The model under review builds one solid part; all positions refer to its coordinate system, in mm. Round coordinates to 2 decimals unless told otherwise and drop trailing zeros. Write each loop counter-clockwise with the first axis right and the second up, starting at its lowest first coordinate (ties: lowest second). Pieces come first, ordered by that corner, then holes.
Item 1: Add section D-D (z = 4.25). Give the boundary of the cut face in (x, y), plus the area to 3 significant figures.
Item 2: Draft analysis for pull direction Y (two halves, no side actions). For faces 1 (the face through (-0.867, -3.905, -2.104)), 2 (the face through (0.61, -2.74, -0.18)), 3 (the face through (2.2, -2.2, 12.7)), state which applies: +Y half, -Y half, draft (parallel to the pull), parting line (faces both ways), or undercut.
Item 3: Add section A-A (y = 0). Give the boundary of the cut face in (x, z) (3 decimals).
Item 4: Clearance check with flat-ended pins moving along their axes: pin 1 Ø1.5 at (y, z) = (4, -7.5) entering from -X; pin 2 Ø4 at (y, z) = (3.5, 2) entering from +X; pin 3 Ø5 at (x, z) = (0.5, 0.5) entering from +Y. State where each tip first meets the part, or that it passes through.
Item 5: To check wall thickness, follow L1, parallel to Y at x = 0, z = 1.5; L2, parallel to Y at x = -2, z = 4.75; L3, parallel to Z at x = 2.75, y = 3.5. State the ranges of each line that lie inside material, in increasing order.
Item 6: Add section C-C (z = 9). Give the boundary of the cut face in (x, y) (3 decimals), plus the area to 3 significant figures.
```python
from build123d import *

# Parameters (mm, degrees)
SKETCH1_R              = 4
BOSS_EXTRUDE1_DEPTH    = 12.7
F_10_CLEARANCE_HOLE1_D = 5.6134
BOSS_EXTRUDE2_START    = -4
SKETCH4_R              = 5.125
SKETCH4_R_2            = 2.8067
BOSS_EXTRUDE2_DEPTH    = 4
FILLET1_R              = 0.5


with BuildPart() as part:
    # Sketch1 → Boss-Extrude1 (new, symmetric)
    with BuildSketch(Plane.XY):
        Circle(SKETCH1_R)
    extrude(amount=BOSS_EXTRUDE1_DEPTH, both=True)

    # #10 Clearance Hole1 (through all)
    with Locations(Plane.XY.offset(12.7)):
        with Locations((0, 0)):
            Hole(F_10_CLEARANCE_HOLE1_D / 2)

    # Sketch4 → Boss-Extrude2 (add)
    with BuildSketch(Plane.XY.offset(12.7).offset(BOSS_EXTRUDE2_START)):
        Circle(SKETCH4_R)
        Circle(SKETCH4_R_2, mode=Mode.SUBTRACT)
    extrude(amount=BOSS_EXTRUDE2_DEPTH)

    # Fillet1
    fillet1_edges = [part.edges().sort_by_distance(p)[0] for p in [
        (-4, 0, 8.7),
    ]]
    fillet(fillet1_edges, radius=FILLET1_R)


solid = part.part
```
Numbers:
1. outline: circle Ø8 at (0, 0); hole circle Ø5.61 at (0, 0)
1. area: 25.5 mm2
2. face 1: parting line
2. face 2: undercut
2. face 3: draft
3. outline: (-5.125, 8.7) - (-4.5, 8.7) arc R0.5 cw to (-4, 8.2) - (-4, -12.7) - (-2.807, -12.7) - (-2.807, 12.7) - (-5.125, 12.7) - close; (2.807, -12.7) - (4, -12.7) - (4, 8.2) arc R0.5 cw to (4.5, 8.7) - (5.125, 8.7) - (5.125, 12.7) - (2.807, 12.7) - close
4. pin 1: stops at x = -2.33
4. pin 2: stops at x = 3.71
4. pin 3: stops at y = 4
5. L1: y = -4 to -2.81, 2.81 to 4
5. L2: y = -3.46 to -1.97, 1.97 to 3.46
5. L3: z = 8.7 to 12.7
6. outline: circle Ø10.25 at (0, 0); hole circle Ø5.613 at (0, 0)
6. area: 57.8 mm2
